from build123d import *
from build123d.topology import SkipClean

# Parameters (mm, degrees)
SKETCH1_R           = 37.5
SKETCH1_R_2         = 3.35
BOSS_EXTRUDE1_DEPTH = 2.5
BOSS_EXTRUDE2_DEPTH = 2.5


with BuildPart() as part:
    # Sketch1 → Boss-Extrude1 (new body)
    with BuildSketch(Plane(origin=(0, 0, 0), x_dir=(1, 0, 0), z_dir=(0, 1, 0))):
        with Locations(Location((0, 0, 0), (0, 0, 270))):
            Circle(SKETCH1_R)
        with Locations(Location((0, 31.5, 0), (0, 0, 270))):
            Circle(SKETCH1_R_2, mode=Mode.SUBTRACT)
        with Locations(Location((27.279800219, -15.75, 0), (0, 0, 270))):
            Circle(SKETCH1_R_2, mode=Mode.SUBTRACT)
        with Locations(Location((-27.279800219, -15.75, 0), (0, 0, 270))):
            Circle(SKETCH1_R_2, mode=Mode.SUBTRACT)
        with BuildLine():
            ThreePointArc((-6.945839996, 28.670634921), (-25.547749412, 14.75), (-28.302418182, -8.320043573))
            ThreePointArc((-28.302418182, -8.320043573), (-20.784609691, -12), (-21.356578186, -20.350591347))
            ThreePointArc((-21.356578186, -20.350591347), (0, -29.5), (21.356578186, -20.350591347))
            ThreePointArc((21.356578186, -20.350591347), (20.784609691, -12), (28.302418182, -8.320043573))
            ThreePointArc((28.302418182, -8.320043573), (25.547749412, 14.75), (6.945839996, 28.670634921))
            ThreePointArc((6.945839996, 28.670634921), (0, 24), (-6.945839996, 28.670634921))
        make_face(mode=Mode.SUBTRACT)
    extrude(amount=BOSS_EXTRUDE1_DEPTH)

    # Sketch2 → Boss-Extrude2 (add)
    with SkipClean():  # the faces are left unmerged after this step: merging them gives an invalid solid
        with BuildSketch(Plane(origin=(0, 0, 0), x_dir=(1, 0, 0), z_dir=(0, 1, 0))):
            with BuildLine():
                Line((-3.5, 31.5), (-3.5, 6.633249581))
                ThreePointArc((-3.5, 6.633249581), (-6.495190528, 3.75), (-7.494562647, -0.285535877))
                Line((-7.494562647, -0.285535877), (-29.029800219, -12.718911087))
                Line((-29.029800219, -12.718911087), (-28.954800219, -12.848814897))
                ThreePointArc((-28.954800219, -12.848814897), (-24.378615117, -14.075), (-25.604800219, -18.651185103))
                Line((-25.604800219, -18.651185103), (-25.529800219, -18.781088913))
                Line((-25.529800219, -18.781088913), (-3.994562647, -6.347713704))
                ThreePointArc((-3.994562647, -6.347713704), (0, -7.5), (3.994562647, -6.347713704))
                Line((3.994562647, -6.347713704), (25.529800219, -18.781088913))
                Line((25.529800219, -18.781088913), (25.604800219, -18.651185103))
                ThreePointArc((25.604800219, -18.651185103), (24.378615117, -14.075), (28.954800219, -12.848814897))
                Line((28.954800219, -12.848814897), (29.029800219, -12.718911087))
                Line((29.029800219, -12.718911087), (7.494562647, -0.285535877))
                ThreePointArc((7.494562647, -0.285535877), (6.495190528, 3.75), (3.5, 6.633249581))
                Line((3.5, 6.633249581), (3.5, 31.5))
                Line((3.5, 31.5), (3.35, 31.5))
                ThreePointArc((3.35, 31.5), (0, 28.15), (-3.35, 31.5))
                Line((-3.35, 31.5), (-3.5, 31.5))
            make_face()
            with BuildLine():
                ThreePointArc((-1.675, 2.901185103), (2.901185103, 1.675), (1.675, -2.901185103))
                ThreePointArc((1.675, -2.901185103), (-2.901185103, -1.675), (-1.675, 2.901185103))
            make_face(mode=Mode.SUBTRACT)
        extrude(amount=BOSS_EXTRUDE2_DEPTH)


solid = part.part
Read the model definition and answer for the solid it produces. Units are mm, in the model's axes. Coordinates: 2 decimals unless noted, no trailing zeros. Write each loop counter-clockwise with the first axis right and the second up, starting at its lowest first coordinate (ties: lowest second). Pieces come first, ordered by that corner, then holes. Notation, with made-up numbers: M -2.75,62 L 40.25,62 A33 cw 40.25,96 Z; hole C 85.25,49 d10. An arc over 180 degrees is marked long. Use a Markdown table: item, result.
Q1. The part is cut by section A-A, the plane x = 0. Write down the section's boundary in (y, z), then the cut area to 3 significant figures.
Answer block:
| item | result |
|---|---|
| outline | M 0,-37.5 L 2.5,-37.5 L 2.5,-34.85 L 0,-34.85 Z; M 0,-28.15 L 2.5,-28.15 L 2.5,-3.35 L 0,-3.35 Z; M 0,3.35 L 2.5,3.35 L 2.5,7.5 L 0,7.5 Z; M 0,29.5 L 2.5,29.5 L 2.5,37.5 L 0,37.5 Z |
| area | 99.0 mm2 |
Q2. The part is cut by section C-C, the plane x = 14.5. Write down the section's boundary in (y, z), then the cut area to 3 significant figures.
Answer block:
| item | result |
|---|---|
| outline | M 0,-34.58 L 2.5,-34.58 L 2.5,-25.69 L 0,-25.69 Z; M 0,4.33 L 2.5,4.33 L 2.5,12.41 L 0,12.41 Z; M 0,25.69 L 2.5,25.69 L 2.5,34.58 L 0,34.58 Z |
| area | 64.7 mm2 |
Q3. The part is cut by section D-D, the plane y = 0.75. Write down the section's boundary in (x, z) (3 decimals), then the cut area to 3 significant figures.
Answer block:
| item | result |
|---|---|
| outline | C 0,0 d75; hole C -27.28,15.75 d6.7; hole M -28.302,8.32 A29.5 ccw -6.946,-28.671 A7.5 cw -3.5,-24.867 L -3.5,-6.633 A7.5 cw -7.495,0.286 L -23.285,9.402 A7.5 cw Z; hole M -21.357,20.351 A7.5 cw -19.785,15.464 L -3.995,6.348 A7.5 cw 3.995,6.348 L 19.785,15.464 A7.5 cw 21.357,20.351 A29.5 ccw Z; hole C 0,-31.5 d6.7; hole C 0,0 d6.7; hole M 3.5,-24.867 A7.5 cw 6.946,-28.671 A29.5 ccw 28.302,8.32 A7.5 cw 23.285,9.402 L 7.495,0.286 A7.5 cw 3.5,-6.633 Z; hole C 27.28,15.75 d6.7 |
| area | 2,240 mm2 |
Q4. Each of these flat-tipped pins is pushed along its axis until it touches: pin 1 Ø0.8 at (y, z) = (1.5, -17) entering from -X; pin 2 Ø1.5 at (x, y) = (-9.5, 2) entering from -Z. Where does it stop, or does it pass through?
Answer block:
| item | result |
|---|---|
| pin 1 | stops at x = -33.63 |
| pin 2 | stops at z = -36.46 |
Q5. Determine the mould class of faces 1 (the face through (-22.818, 1.232, -29.759)), 2 (the face through (1, 0, -9)), 3 (the face through (-0.1, 1.2, 7.5)) for opening direction Z: released by +Z, released by -Z, zero draft, split by the parting line, or undercut.
Answer block:
| item | result |
|---|---|
| face 1 | split by the parting line |
| face 2 | zero draft |
| face 3 | undercut |
Q6. The part is cut by section B-B, the plane z = -31.5. Write down the section's boundary in (x, y), then the cut area to 3 significant figures.
Answer block:
| item | result |
|---|---|
| outline | M -20.35,0 L -3.35,0 L -3.35,2.5 L -20.35,2.5 Z; M 3.35,0 L 20.35,0 L 20.35,2.5 L 3.35,2.5 Z |
| area | 85.0 mm2 |
Q7. Straight lines are drawn through the part: L1, parallel to X at y = 1.8, z = 13.5; L2, parallel to Z at x = -6, y = 2.1; L3, parallel to X at y = 1, z = -10. For each, find the intervals that lie inside material, in ascending order. Write a range as [from, to].
Answer block:
| item | result |
|---|---|
| L1 | x = [-34.99, -29.76], [-24.8, -16.38], [16.38, 24.8], [29.76, 34.99] |
| L2 | z = [-37.02, -27], [-4.5, 7.51], [28.88, 37.02] |
| L3 | x = [-36.14, -27.75], [-3.5, 3.5], [27.75, 36.14] |
